Part print with two shaded views. Sizes in mm from the minimum x, y, z corner. A direction names the side the tool comes from. Round coordinates to 2 decimals unless told otherwise and drop trailing zeros. Order: outer loops, then holes, each group sorted by start corner. A loop starts at its lowest first (then second) coordinate and runs counter-clockwise, first axis right, second up. Notation, with made-up numbers: (85.5, 12.5) - (104.5, 12.5) arc R20 cw to (104.5, 38.5) - close; hole circle Ø10 at (-20.5, -32.5). An arc over 180 degrees is marked (long way). Answer as CSV lines item,"result". Start each with the question number.
1. Pin check, flat tips, straight feed: pin 1 Ø6 at (y, z) = (11, 25) entering from +X; pin 2 Ø16 at (y, z) = (24.5, 14) entering from +X; pin 3 Ø6 at (y, z) = (15.5, 14) entering from -X; pin 4 Ø5 at (x, y) = (23.5, 14) entering from +Z. Stop position of each tip, or through.
2. Band-saw the part on C-C on x = 16. List the corners of the cut face in (y, z), then the cut area to 3 significant figures.
3. 3-axis set-ups, long thin cutter, end or side, ignore diameter. For the marked faces 4, 5 and 6: which of +Z, -Z, +X, -X, +Y, -Y reach the whole face in a straight line?
4. Band-saw the part on D-D on y = 25.25. List the corners of the cut face in (x, z), then the cut area to 3 significant figures.
5. Band-saw the part on A-A on z = 15. List the corners of the cut face in (x, y).
6. Wall check: line 1 along Y through (x, z) = (12.85, 15); line 2 along X through (y, z) = (15, 15); line 3 along Y through (x, z) = (41, 27). Give the ranges that are in metal, low to high. Write a range as [from, to].
7. Pull direction X, two halves, no side cores. Call the marked faces 1, 2 and 3: released by +X, released by -X, zero draft, split by the parting line, or undercut.
8. Band-saw the part on B-B on y = 13.75. List the corners of the cut face in (x, z), then the cut area to 3 significant figures.
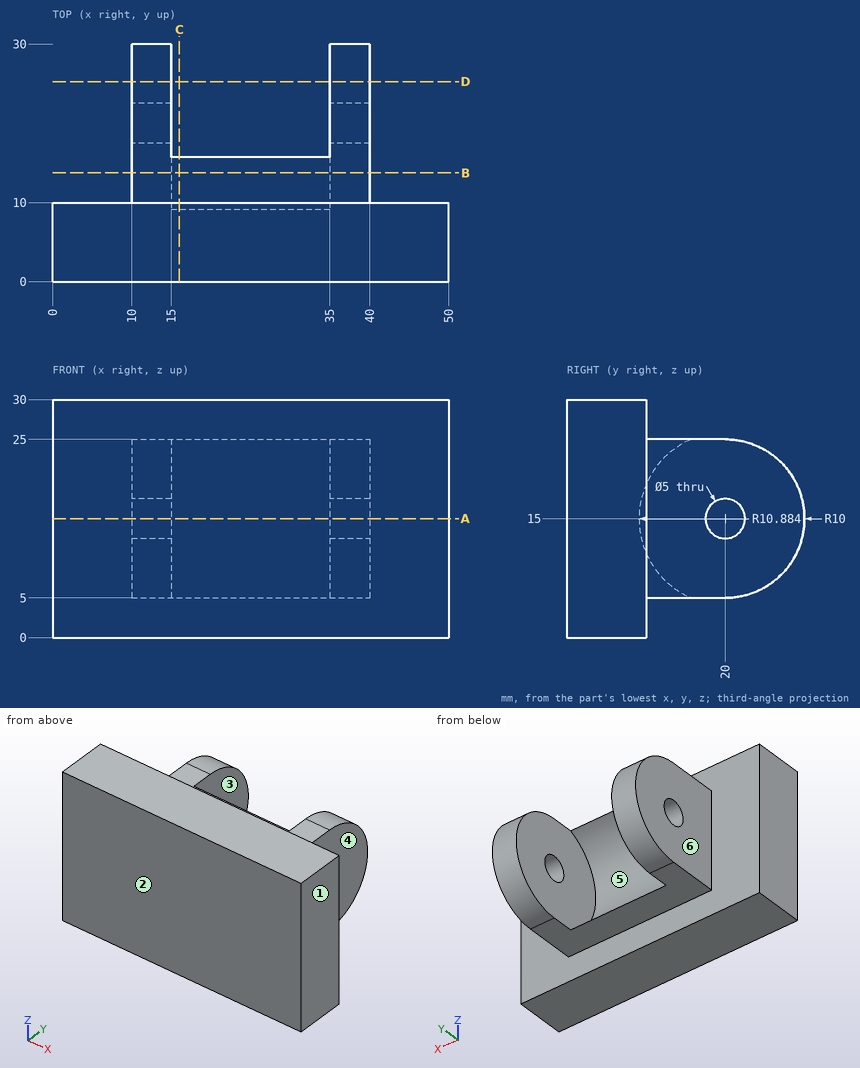
Reply:
1,pin 1,"stops at x = 50"
1,pin 2,"stops at x = 40"
1,pin 3,"stops at x = 10"
1,pin 4,"stops at z = 25"
2,outline,"(0, 0) - (10, 0) - (10, 5) - (15.7, 5) arc R10.88 cw to (15.7, 25) - (10, 25) - (10, 30) - (0, 30) - close"
2,area,"319 mm2"
3,face 4,"+Z, -Z, +X, +Y"
3,face 5,"+Y"
3,face 6,"+Z, -Z, -X, +Y"
4,outline,"(10, 6.49) - (15, 6.49) - (15, 23.51) - (10, 23.51) - close; (35, 6.49) - (40, 6.49) - (40, 23.51) - (35, 23.51) - close"
4,area,"170 mm2"
5,outline,"(0, 0) - (50, 0) - (50, 10) - (40, 10) - (40, 17.5) - (35, 17.5) - (35, 9.12) - (15, 9.12) - (15, 17.5) - (10, 17.5) - (10, 10) - (0, 10) - close; (10, 22.5) - (15, 22.5) - (15, 30) - (10, 30) - close; (35, 22.5) - (40, 22.5) - (40, 30) - (35, 30) - close"
6,line 1,"y = [0, 17.5], [22.5, 30]"
6,line 2,"x = [10, 15], [35, 40]"
6,line 3,"y = [0, 10]"
7,face 1,"released by +X"
7,face 2,"zero draft"
7,face 3,"undercut"
8,outline,"(10, 5) - (40, 5) - (40, 25) - (10, 25) - close; hole (15, 6.09) - (35, 6.09) - (35, 23.91) - (15, 23.91) - close"
8,area,"244 mm2"
